The figure shows three views and two pictorial views of one solid part (mm, origin at its lowest corner). Answer the questions. Give positions to 0.01 mm unless a question says otherwise; leave off trailing zeros. Loops run counter-clockwise (first coordinate to the right, second up) from the corner with the lowest first, then second, coordinate; pieces in that order, holes last. Notation, with made-up numbers: (46, 6) - (86, 6) arc R10 ccw to (86, 20) - close; hole circle Ø2 at (-29, 39). An arc over 180 degrees is marked (long way). Use a Markdown table: item, result. Add a question column.
Item 1: Consider probe 1 along Z at (x, y) = (22.5, 1.55); probe 2 along Z at (x, y) = (19, 2.05); probe 3 along X at (y, z) = (1.65, 146.15). Determine where each line is inside the solid, lowest interval first. Write a range as [from, to].
Item 2: A cutting plane is placed at D-D (x = 48). Determine the outline of the cut face in (y, z) (3 decimals).
Item 3: A cutting plane is placed at A-A (z = 123.5). Determine the outline of the cut face in (x, y) (3 decimals), plus the area to 3 significant figures.
Item 4: This flat-tipped pin is pushed along its axis until it touches: P1, Ø1, axis at x = 22.5, z = 146.15, coming from the +Y side. Where does it stop, or does it pass through?
Item 5: A cutting plane is placed at C-C (z = 10). Determine the outline of the cut face in (x, y) (3 decimals), plus the area to 3 significant figures.
Item 6: A cutting plane is placed at B-B (y = 2.55). Determine the outline of the cut face in (x, z).
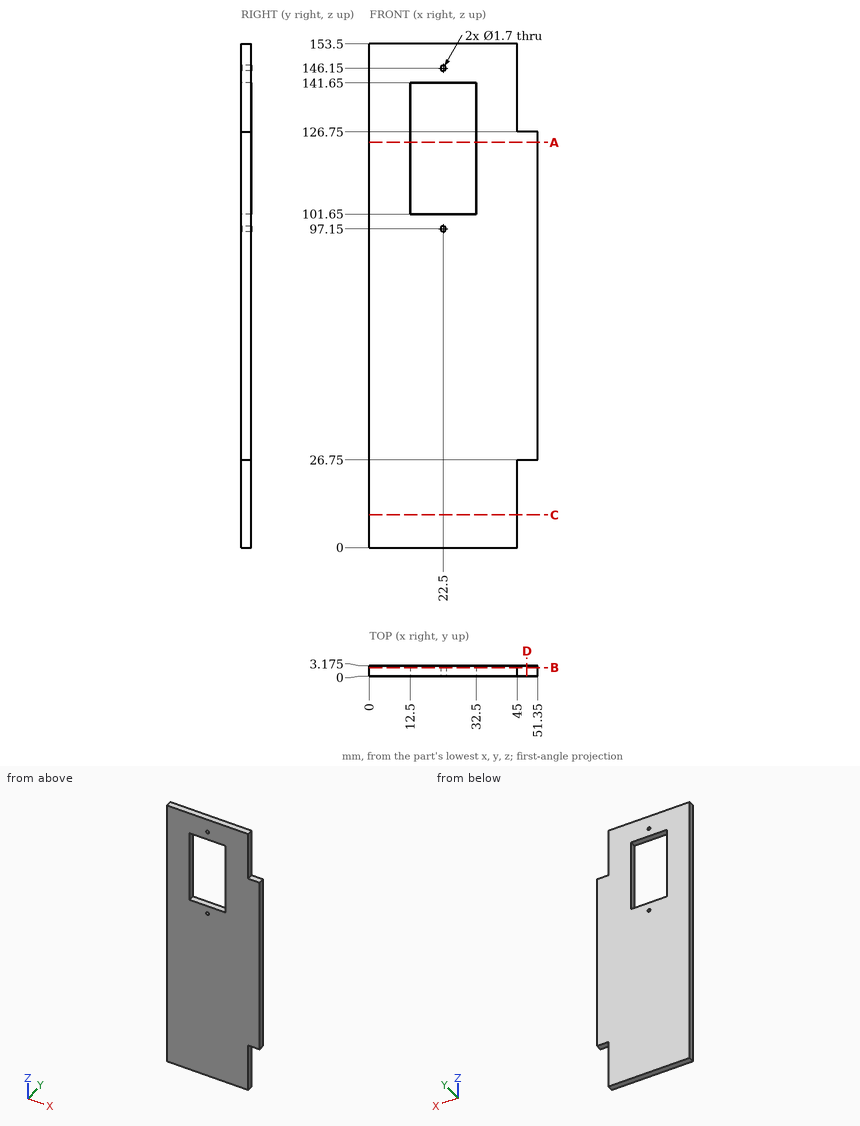
Geometry says:
| question | item | result |
|---|---|---|
| 1 | probe 1 | [0, 96.3], [98, 101.65], [141.65, 145.3], [147, 153.5] |
| 1 | probe 2 | [0, 101.65], [141.65, 153.5] |
| 1 | probe 3 | [0, 21.65], [23.35, 45] |
| 2 | outline | (0, 26.75) - (3.175, 26.75) - (3.175, 126.75) - (0, 126.75) - close |
| 3 | outline | (0, 0) - (12.5, 0) - (12.5, 3.175) - (0, 3.175) - close; (32.5, 0) - (51.35, 0) - (51.35, 3.175) - (32.5, 3.175) - close |
| 3 | area | 99.5 mm² |
| 4 | P1 | through |
| 5 | outline | (0, 0) - (45, 0) - (45, 3.175) - (0, 3.175) - close |
| 5 | area | 143 mm² |
| 6 | outline | (0, 0) - (45, 0) - (45, 26.75) - (51.35, 26.75) - (51.35, 126.75) - (45, 126.75) - (45, 153.5) - (0, 153.5) - close; hole (12.5, 101.65) - (32.5, 101.65) - (32.5, 141.65) - (12.5, 141.65) - close; hole circle Ø1.7 at (22.5, 97.15); hole circle Ø1.7 at (22.5, 146.15) |
